Geometry check sheet. Reference: the model listing, model coordinates, mm. A direction names the side the tool comes from. Coordinates: 2 decimals unless noted, no trailing zeros. Write each loop counter-clockwise with the first axis right and the second up, starting at its lowest first coordinate (ties: lowest second). Pieces come first, ordered by that corner, then holes. Notation, with made-up numbers: (75, 66) -> (108, 66) arc R25 ccw to (108, 78) -> close; hole circle Ø11 at (13.25, 89.25). An arc over 180 degrees is marked (long way). Answer in a Markdown table with one row per item. Add a question column.
1. Cross-section at C-C on z = -2.5. Record the cut outline in (x, y).
2. Cross-section at D-D on y = 24. Record the cut outline in (x, z), and give its area (3 significant figures).
3. Cross-section at A-A on x = 0. Record the cut outline in (y, z).
4. Depth check by flat-ended pin: P1, Ø8, axis at y = 10.5, z = 6, coming from the +X side; P2, Ø5, axis at y = 35.5, z = 20, coming from the -X side; P3, Ø2, axis at x = 16.5, y = 25.5, coming from the -Z side; P4, Ø8, axis at x = 33.5, z = 28.5, coming from the -Y side. Enter the tip coordinate at first touch or a pass-through.
5. Set-up check for faces 4 (the cylindrical face through (-5.506, 43.327, 24.796)), 5 (the cylindrical face through (-6.883, 21.448, 30.995)), 6 (the cylindrical face through (0.33, 2.5, -40.64)), 7 (the flat face through (12.065, 3, 66)): record each of +Z, -Z, +X, -X, +Y, -Y from which the full face is reachable in a straight line by a thin tool's end or side.
6. Scan lines: L1, parallel to Y at x = -35, z = -6; L2, parallel to Y at x = 10, z = 62.5; L3, parallel to X at y = 17.5, z = 0. Record each from-to range of solid material in increasing order. Write a range as from..to.
7. Cross-section at B-B on y = 41. Record the cut outline in (x, z), and give its area (3 significant figures).
8. Mould release check, pull along Y, two halves, no side actions. Record for faces 1 (the flat face through (0, 51.054, 0)), 2 (the flat face through (-12.065, 3, 66)), 3 (the cylindrical face through (-28.547, 8.211, -0.621)): pulls with the +Y half, pulls with the -Y half, needs draft (parallel to the pull), parting line crosses it, or undercut.
```python
from build123d import *

# Parameters (mm, degrees)
BOSS_EXTRUDE1_DEPTH = 5.08
FILLET1_R           = 12.7
FILLET2_R           = 12.7
SKETCH2_R           = 28.575
BOSS_EXTRUDE2_DEPTH = 6.35
SKETCH3_R           = 31.75
BOSS_EXTRUDE3_DEPTH = 20.32
SKETCH4_R           = 38.1
BOSS_EXTRUDE4_DEPTH = 4.064
SKETCH5_R           = 25.4
BOSS_EXTRUDE5_DEPTH = 15.24


with BuildPart() as part:
    # Sketch1 → Boss-Extrude1 (new body)
    with BuildSketch(Plane(origin=(0, 0, 0), x_dir=(1, 0, 0), z_dir=(0, 1, 0))):
        with BuildLine():
            Line((51.054, -2.54), (51.054, 0))
            Line((51.054, 0), (51.054, 25.4))
            add(Edge.make_bspline(
                [(51.054, 25.4), (35.593374206, 25.086699202), (25.873960254, 31.339237081)],
                knots=[0, 0, 0, 0.413959763, 0.413959763, 0.413959763], degree=2))
            add(Edge.make_bspline(
                [(25.873960254, 31.339237081), (24.125496917, 32.46403054), (22.562829629, 33.80130647)],
                knots=[0.413959763, 0.413959763, 0.413959763, 0.488428602, 0.488428602, 0.488428602], degree=2))
            ThreePointArc((22.562829629, 33.80130647), (0, 40.64), (-22.562829629, 33.80130647))
            add(Edge.make_bspline(
                [(-25.873960254, 31.339237081), (-24.125496917, 32.46403054), (-22.562829629, 33.80130647)],
                knots=[0.413959763, 0.413959763, 0.413959763, 0.488428602, 0.488428602, 0.488428602], degree=2))
            add(Edge.make_bspline(
                [(-51.054, 25.4), (-35.593374206, 25.086699202), (-25.873960254, 31.339237081)],
                knots=[0, 0, 0, 0.413959763, 0.413959763, 0.413959763], degree=2))
            Line((-51.054, 25.4), (-51.054, 0))
            Line((-51.054, 0), (-51.054, -2.54))
            add(Edge.make_bspline(
                [(-51.054, -2.54), (-42.130232366, -11.547896864), (-34.503914612, -21.472994119)],
                knots=[0, 0, 0, 0.367111941, 0.367111941, 0.367111941], degree=2))
            add(Edge.make_bspline(
                [(-34.503914612, -21.472994119), (-32.482868864, -24.103237999), (-30.552942986, -26.797896838)],
                knots=[0.367111941, 0.367111941, 0.367111941, 0.46440005, 0.46440005, 0.46440005], degree=2))
            add(Edge.make_bspline(
                [(-30.552942986, -26.797896838), (-19.928127461, -41.632794577), (-12.065, -58.42)],
                knots=[0.46440005, 0.46440005, 0.46440005, 1, 1, 1], degree=2))
            Line((-12.065, -58.42), (-12.065, -71.12))
            Line((-12.065, -71.12), (12.065, -71.12))
            Line((12.065, -71.12), (12.065, -58.42))
            add(Edge.make_bspline(
                [(30.552942986, -26.797896838), (19.928127461, -41.632794577), (12.065, -58.42)],
                knots=[0.46440005, 0.46440005, 0.46440005, 1, 1, 1], degree=2))
            add(Edge.make_bspline(
                [(34.503914612, -21.472994119), (32.482868864, -24.103237999), (30.552942986, -26.797896838)],
                knots=[0.367111941, 0.367111941, 0.367111941, 0.46440005, 0.46440005, 0.46440005], degree=2))
            add(Edge.make_bspline(
                [(51.054, -2.54), (42.130232366, -11.547896864), (34.503914612, -21.472994119)],
                knots=[0, 0, 0, 0.367111941, 0.367111941, 0.367111941], degree=2))
        make_face()
    extrude(amount=BOSS_EXTRUDE1_DEPTH)

    # Fillet1
    fillet1_edges = [part.edges().sort_by_distance(p)[0] for p in [
        (-12.065, 2.54, 58.42),
    ]]
    fillet(fillet1_edges, radius=FILLET1_R)

    # Fillet2
    fillet2_edges = [part.edges().sort_by_distance(p)[0] for p in [
        (12.065, 2.54, 58.42),
    ]]
    fillet(fillet2_edges, radius=FILLET2_R)

    # Sketch2 → Boss-Extrude2 (add)
    with BuildSketch(Plane(origin=(0, 5.08, 0), x_dir=(1, 0, 0), z_dir=(0, 1, 0))):
        with Locations((0, -0.635)):
            Circle(SKETCH2_R)
    extrude(amount=BOSS_EXTRUDE2_DEPTH)

    # Sketch3 → Boss-Extrude3 (add)
    with BuildSketch(Plane(origin=(0, 11.43, 0), x_dir=(1, 0, 0), z_dir=(0, 1, 0))):
        Circle(SKETCH3_R)
    extrude(amount=BOSS_EXTRUDE3_DEPTH)

    # Sketch4 → Boss-Extrude4 (add)
    with BuildSketch(Plane(origin=(0, 31.75, 0), x_dir=(1, 0, 0), z_dir=(0, 1, 0))):
        Circle(SKETCH4_R)
    extrude(amount=BOSS_EXTRUDE4_DEPTH)

    # Sketch5 → Boss-Extrude5 (add)
    with BuildSketch(Plane(origin=(0, 35.814, 0), x_dir=(1, 0, 0), z_dir=(0, 1, 0))):
        Circle(SKETCH5_R)
    extrude(amount=BOSS_EXTRUDE5_DEPTH)


solid = part.part
```
Results found:
| question | item | result |
|---|---|---|
| 1 | outline | (-51.05, 0) -> (51.05, 0) -> (51.05, 5.08) -> (28.4, 5.08) -> (28.4, 11.43) -> (31.65, 11.43) -> (31.65, 31.75) -> (38.02, 31.75) -> (38.02, 35.81) -> (25.28, 35.81) -> (25.28, 51.05) -> (-25.28, 51.05) -> (-25.28, 35.81) -> (-38.02, 35.81) -> (-38.02, 31.75) -> (-31.65, 31.75) -> (-31.65, 11.43) -> (-28.4, 11.43) -> (-28.4, 5.08) -> (-51.05, 5.08) -> close |
| 2 | outline | circle Ø63.5 at (0, 0) |
| 2 | area | 3,170 mm^2 |
| 3 | outline | (0, -40.64) -> (5.08, -40.64) -> (5.08, -27.94) -> (11.43, -27.94) -> (11.43, -31.75) -> (31.75, -31.75) -> (31.75, -38.1) -> (35.81, -38.1) -> (35.81, -25.4) -> (51.05, -25.4) -> (51.05, 25.4) -> (35.81, 25.4) -> (35.81, 38.1) -> (31.75, 38.1) -> (31.75, 31.75) -> (11.43, 31.75) -> (11.43, 29.21) -> (5.08, 29.21) -> (5.08, 71.12) -> (0, 71.12) -> close |
| 4 | P1 | stops at x = 31.68 |
| 4 | P2 | stops at x = -33.84 |
| 4 | P3 | stops at z = -27.71 |
| 4 | P4 | stops at y = 0 |
| 5 | face 4 | +Y |
| 5 | face 5 | none |
| 5 | face 6 | -Z, +Y, -Y |
| 5 | face 7 | +Z, +X, +Y, -Y |
| 6 | L1 | y = 0..5.08, 31.75..35.81 |
| 6 | L2 | y = 0..5.08 |
| 6 | L3 | x = -31.75..31.75 |
| 7 | outline | circle Ø50.8 at (0, 0) |
| 7 | area | 2,030 mm^2 |
| 8 | face 1 | pulls with the +Y half |
| 8 | face 2 | needs draft |
| 8 | face 3 | undercut |
